from build123d import *

# Parameters (mm, degrees)
SKETCH2_R           = 15
BOSS_EXTRUDE2_DEPTH = 5
SKETCH3_W           = 50
SKETCH3_H           = 5
BOSS_EXTRUDE3_DEPTH = 60
SKETCH4_R           = 10
BOSS_EXTRUDE4_DEPTH = 15
SKETCH5_W           = 50
SKETCH5_H           = 70
SKETCH5_R           = 15
BOSS_EXTRUDE5_DEPTH = 7


with BuildPart() as part:
    # Sketch2 → Boss-Extrude2 (new, symmetric)
    with BuildSketch(Plane.XY.offset(30)):
        with BuildLine():
            Line((-25, 22.5), (-25, -22.5))
            Line((-25, -22.5), (25, -22.5))
            Line((25, -22.5), (25, 22.5))
            ThreePointArc((25, 22.5), (0, 47.5), (-25, 22.5))
        make_face()
        with Locations((0, 22.5)):
            Circle(SKETCH2_R, mode=Mode.SUBTRACT)
    boss_extrude2 = extrude(amount=BOSS_EXTRUDE2_DEPTH, both=True)

    # Sketch3 → Boss-Extrude3 (add)
    with BuildSketch(Plane(origin=(0, 0, 25), x_dir=(-1, 0, 0), z_dir=(0, 0, -1))):
        with Locations((0, -20)):
            Rectangle(SKETCH3_W, SKETCH3_H)
    extrude(amount=BOSS_EXTRUDE3_DEPTH)

    # Mirror3: Boss-Extrude2 across plane
    add(boss_extrude2.mirror(Plane.XY))

    # Sketch4 → Boss-Extrude4 (add)
    with BuildSketch(Plane.XZ.offset(22.5)):
        with Locations(Location((0, 0, 0), (0, 0, 270))):
            Circle(SKETCH4_R)
    extrude(amount=BOSS_EXTRUDE4_DEPTH)

    # Sketch5 → Boss-Extrude5 (add)
    with BuildSketch(Plane.XZ.offset(22.5)):
        Rectangle(SKETCH5_W, SKETCH5_H)
        with Locations(Location((0, 0, 0), (0, 0, 270))):
            Circle(SKETCH5_R, mode=Mode.SUBTRACT)
    extrude(amount=BOSS_EXTRUDE5_DEPTH)


solid = part.part
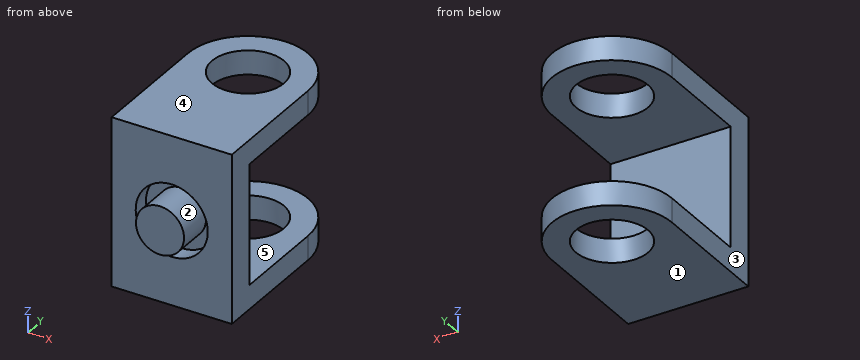
Work out the finished part from the listing and answer in its coordinate system (mm). Face numbers are marked on the shaded views. A direction names the side the tool comes from. Round coordinates to 2 decimals unless told otherwise and drop trailing zeros. Write each loop counter-clockwise with the first axis right and the second up, starting at its lowest first coordinate (ties: lowest second). Pieces come first, ordered by that corner, then holes. Notation, with made-up numbers: (51.5, 55) -> (67.5, 55) arc R16 cw to (67.5, 80) -> close; hole circle Ø2 at (35, 43). An arc over 180 degrees is marked (long way). Answer as CSV lines item,"result". Start each with the question number.
(1) Each of these flat-tipped pins is pushed along its axis until it touches: pin 1 (15 mm diameter, centred on x = -3.5, y = 11, fed in from -Z); pin 2 (1 mm diameter, centred on x = 11, z = -26, fed in from +Y); pin 3 (2 mm diameter, centred on x = 0, z = -16, fed in from -Y); pin 4 (18 mm diameter, centred on x = 0, y = 22.5, fed in from -Z). Where does it stop, or does it pass through?
(2) The part is cut by section D-D, the plane y = 31. Give the vertices of the cut face in (x, z).
(3) The part is cut by section B-B, the plane z = 0. Give the vertices of the cut face in (x, y), then the cut area to 3 significant figures.
(4) A tool of negligible diameter and unlimited length cuts with its end or side. For the marked faces 4 and 5, from which of +Z, -Z, +X, -X, +Y, -Y can it reach the whole face along a straight path? Write none if from no direction.
(5) The mould has two halves that part along Z. Classify the marked faces 1, 2 and 3: +Z half, -Z half, draft (parallel to the pull), parting line (faces both ways), or undercut.
(6) Find the intervals of material crossed by probe 1 along Z at (x, y) = (-14, -7); probe 2 along Y at (x, z) = (0, -30.75); probe 3 along X at (y, z) = (22, -31), in increasing order.
(7) The part is cut by section A-A, the plane x = 0. Give the vertices of the cut face in (y, z), then the cut area to 3 significant figures.
(8) The part is cut by section C-C, the plane y = 40. Give the vertices of the cut face in (x, z).
Output values:
1,pin 1,"stops at z = -35"
1,pin 2,"stops at y = 45.19"
1,pin 3,"stops at y = -29.5"
1,pin 4,"passes through"
2,outline,"(-23.51, -35) -> (-12.36, -35) -> (-12.36, -25) -> (-23.51, -25) -> close; (-23.51, 25) -> (-12.36, 25) -> (-12.36, 35) -> (-23.51, 35) -> close; (12.36, -35) -> (23.51, -35) -> (23.51, -25) -> (12.36, -25) -> close; (12.36, 25) -> (23.51, 25) -> (23.51, 35) -> (12.36, 35) -> close"
3,outline,"(-25, -29.5) -> (-15, -29.5) -> (-15, -22.5) -> (-10, -22.5) -> (-10, -37.5) -> (10, -37.5) -> (10, -22.5) -> (15, -22.5) -> (15, -29.5) -> (25, -29.5) -> (25, -17.5) -> (-25, -17.5) -> close"
3,area,"690 mm²"
4,face 4,"+Z, +X, -X, +Y, -Y"
4,face 5,"+X, -X, +Y"
5,face 1,"-Z half"
5,face 2,"undercut"
5,face 3,"draft"
6,probe 1,"z = -35 to -25, 25 to 35"
6,probe 2,"y = -29.5 to 7.5, 37.5 to 47.5"
6,probe 3,"x = -25 to -14.99, 14.99 to 25"
7,outline,"(-37.5, -10) -> (-22.5, -10) -> (-22.5, -15) -> (-29.5, -15) -> (-29.5, -35) -> (7.5, -35) -> (7.5, -25) -> (-17.5, -25) -> (-17.5, 25) -> (7.5, 25) -> (7.5, 35) -> (-29.5, 35) -> (-29.5, 15) -> (-22.5, 15) -> (-22.5, 10) -> (-37.5, 10) -> close; (37.5, -35) -> (47.5, -35) -> (47.5, -25) -> (37.5, -25) -> close; (37.5, 25) -> (47.5, 25) -> (47.5, 35) -> (37.5, 35) -> close"
7,area,"1,630 mm²"
8,outline,"(-17.85, -35) -> (17.85, -35) -> (17.85, -25) -> (-17.85, -25) -> close; (-17.85, 25) -> (17.85, 25) -> (17.85, 35) -> (-17.85, 35) -> close"
